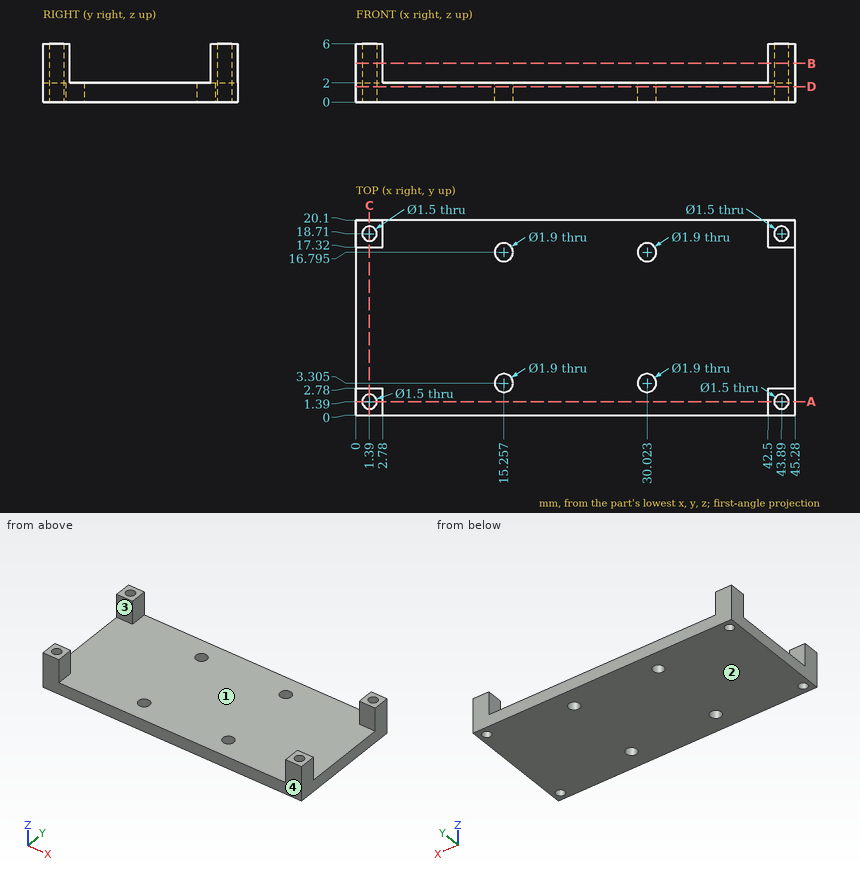
Can you work these out from the drawing? Everything is in mm from the part's minimum corner. A direction names the side the tool comes from. Round coordinates to 2 decimals unless told otherwise and drop trailing zeros. Write each loop counter-clockwise with the first axis right and the second up, starting at its lowest first coordinate (ties: lowest second). Pieces come first, ordered by that corner, then holes. Notation, with made-up numbers: (-23, 84.5) - (-11, 84.5) arc R30 ccw to (-11, 118.5) - close; hole circle Ø9 at (-20.5, 88). An arc over 180 degrees is marked (long way). Write each question's results on one line, items separated by ' | '. Start each with the question number.
1) Which directions (+Z, -Z, +X, -X, +Y, -Y) give clear straight access to the entire face, cutting with the end or side of a thin tool? Please do the marked faces 3 and 4.
2) Suppose I cut it at D-D (z = 1.6). Give the number of separate pieces and of enclosed holes in the cut face, and give its area (3 significant figures).
3) Suppose I cut it at B-B (z = 4). List the corners of the cut face in (x, y) for me.
4) Suppose I cut it at A-A (y = 1.39). List the corners of the cut face in (x, z) for me.
5) We'd pull the mould along X, two halves only. Please class the marked faces 1 and 2: released by +X, released by -X, zero draft, split by the parting line, or undercut.
6) For pin 1 Ø1.5 at (x, z) = (36, 3) entering from -Y, with a flat end and sliding along its axis, tell me the tip position at first contact or that it passes through.
7) Please list where these lines run through material, in increasing order: line 1 (Y direction, x = 1.39, z = 2.65); line 2 (X direction, y = 1.5, z = 4.6); line 3 (Y direction, x = 1.39, z = 1.4).
8) Suppose I cut it at C-C (x = 1.39). List the corners of the cut face in (y, z) for me.
Here are the results:
1) face 3: +Z, +X, -X | face 4: +Z, -Z, +X, -X, -Y
2) separate pieces: 1 | enclosed holes: 8 | area: 892 mm2
3) outline: (0, 0) - (2.78, 0) - (2.78, 2.78) - (0, 2.78) - close; (0, 17.32) - (2.78, 17.32) - (2.78, 20.1) - (0, 20.1) - close; (42.5, 0) - (45.28, 0) - (45.28, 2.78) - (42.5, 2.78) - close; (42.5, 17.32) - (45.28, 17.32) - (45.28, 20.1) - (42.5, 20.1) - close; hole circle Ø1.5 at (1.39, 1.39); hole circle Ø1.5 at (1.39, 18.71); hole circle Ø1.5 at (43.89, 1.39); hole circle Ø1.5 at (43.89, 18.71)
4) outline: (0, 0) - (0.64, 0) - (0.64, 6) - (0, 6) - close; (2.14, 0) - (43.14, 0) - (43.14, 6) - (42.5, 6) - (42.5, 2) - (2.78, 2) - (2.78, 6) - (2.14, 6) - close; (44.64, 0) - (45.28, 0) - (45.28, 6) - (44.64, 6) - close
5) face 1: undercut | face 2: zero draft
6) pin 1: passes through
7) line 1: y = 0 to 0.64, 2.14 to 2.78, 17.32 to 17.96, 19.46 to 20.1 | line 2: x = 0 to 0.65, 2.13 to 2.78, 42.5 to 43.15, 44.63 to 45.28 | line 3: y = 0 to 0.64, 2.14 to 17.96, 19.46 to 20.1
8) outline: (0, 0) - (0.64, 0) - (0.64, 6) - (0, 6) - close; (2.14, 0) - (17.96, 0) - (17.96, 6) - (17.32, 6) - (17.32, 2) - (2.78, 2) - (2.78, 6) - (2.14, 6) - close; (19.46, 0) - (20.1, 0) - (20.1, 6) - (19.46, 6) - close
